from build123d import *

# Parameters (mm, degrees)
F1_DEPTH = 25
F2_DEPTH = 25
F3_R     = 10.5
F4_DEPTH = 25
F6_DEPTH = 25


with BuildPart() as f1:
    # F0 (on Top) → F1 (new body)
    with BuildSketch(Plane.XY):
        with BuildLine():
            Line((-7.459, 75), (-15, 75))
            Line((-15, 75), (-15, 15))
            ThreePointArc((-15, 15), (-16.614759, 6.882058), (-21.213203, 0))
            Line((-21.213203, 0), (-63.534251, -42.321048))
            Line((-63.534251, -42.321048), (-58.201959, -47.65334))
            Line((-58.201959, -47.65334), (-21.537765, -10.989146))
            Line((-21.537765, -10.989146), (-10.989146, -21.537765))
            Line((-10.989146, -21.537765), (-47.65334, -58.201959))
            Line((-47.65334, -58.201959), (-42.321048, -63.534251))
            Line((-42.321048, -63.534251), (0, -21.213203))
            Line((0, -21.213203), (42.321048, -63.534251))
            Line((42.321048, -63.534251), (47.65334, -58.201959))
            Line((47.65334, -58.201959), (10.989146, -21.537765))
            Line((10.989146, -21.537765), (21.537765, -10.989146))
            Line((21.537765, -10.989146), (58.201959, -47.65334))
            Line((58.201959, -47.65334), (63.534251, -42.321048))
            Line((63.534251, -42.321048), (21.213203, 0))
            ThreePointArc((21.213203, 0), (16.614759, 6.882058), (15, 15))
            Line((15, 15), (15, 75))
            Line((15, 75), (7.459, 75))
            Line((7.459, 75), (7.459, 23.149))
            Line((7.459, 23.149), (-7.459, 23.149))
            Line((-7.459, 23.149), (-7.459, 75))
        make_face()
    extrude(amount=F1_DEPTH)

    # F0 (on Top) → F2 (join)
    with BuildSketch(Plane.XY):
        with BuildLine():
            Line((-15, 15), (-15, 75))
            ThreePointArc((-15, 75), (-36.186316, 15.064984), (-63.534251, -42.321048))
            Line((-63.534251, -42.321048), (-21.213203, 0))
            ThreePointArc((-21.213203, 0), (-16.614759, 6.882058), (-15, 15))
        make_face()
        with BuildLine():
            ThreePointArc((63.534251, -42.321048), (36.207052, 15.073562), (15, 75))
            Line((15, 75), (15, 15))
            ThreePointArc((15, 15), (16.614759, 6.882058), (21.213203, 0))
            Line((21.213203, 0), (63.534251, -42.321048))
        make_face()
        with BuildLine():
            Line((0, -21.213203), (-42.321048, -63.534251))
            ThreePointArc((-42.321048, -63.534251), (0, -52.921768), (42.321048, -63.534251))
            Line((42.321048, -63.534251), (0, -21.213203))
        make_face()
    extrude(amount=F2_DEPTH)

    # F3 (on face) → F4 (cut)
    with BuildSketch(Plane.XY.offset(25)):
        Circle(F3_R)
    extrude(amount=-F4_DEPTH, mode=Mode.SUBTRACT)

    # F5 (on face) → F6 (cut)
    with BuildSketch(Plane.XY.offset(25)):
        with BuildLine():
            ThreePointArc((-15.367649, 53.450763), (-29.148649, 12.456713), (-47.984254, -26.474612))
            Line((-47.984254, -26.474612), (-21.509642, 0))
            ThreePointArc((-21.509642, 0), (-16.96133, 6.99149), (-15.367649, 15.178569))
            Line((-15.367649, 15.178569), (-15.367649, 53.450763))
        make_face()
        with BuildLine():
            ThreePointArc((-28.007545, -49.472019), (0.463168, -44.355391), (28.851137, -49.912784))
            Line((28.851137, -49.912784), (0, -21.263063))
            Line((0, -21.263063), (-28.007545, -49.472019))
        make_face()
        with BuildLine():
            ThreePointArc((47.949795, -26.474612), (29.787416, 12.835137), (14.770781, 53.450763))
            Line((14.770781, 53.450763), (14.770781, 15.619874))
            ThreePointArc((14.770781, 15.619874), (16.322077, 7.253759), (20.769704, 0))
            Line((20.769704, 0), (47.949795, -26.474612))
        make_face()
    extrude(amount=-F6_DEPTH, mode=Mode.SUBTRACT)


solid = f1.part
Geometry check sheet. Reference: the model listing, model coordinates, mm. A direction names the side the tool comes from. Give positions to 0.01 mm unless a question says otherwise; leave off trailing zeros. Order: outer loops, then holes, each group sorted by start corner. A loop starts at its lowest first (then second) coordinate and runs counter-clockwise, first axis right, second up. Notation, with made-up numbers: M 65.25,59 L 92.25,59 A17 ccw 92.25,89 Z; hole C 78.5,53.5 d3. An arc over 180 degrees is marked long. Use a Markdown table: item, result.
Item 1: Material ranges on line 1 along Y through (x, z) = (0, 11.5); line 2 along X through (y, z) = (-6, 18); line 3 along X through (y, z) = (-37, 3.75), recorded low to high.
Answers follow:
| item | result |
|---|---|
| line 1 | y = -52.92 to -44.35, -21.26 to -10.5, 10.5 to 23.15 |
| line 2 | x = -45.37 to -37.32, -27.51 to -8.62, 8.62 to 26.93, 38.02 to 45.39 |
| line 3 | x = -60.68 to -47.55, -26.45 to -15.62, 15.85 to 26.45, 47.55 to 60.69 |
Item 2: Tool access check on faces 4 (the flat face through (0, 23.149, 12)), 5 (the cylindrical face through (16.279, 7.366, 12.675)), 6 (the flat face through (60.831, -45.025, 12.325)). Record the directions out of +Z, -Z, +X, -X, +Y, -Y that give a thin tool (end or side, any length) a straight path to the whole face; none if there is none.
Answers follow:
| item | result |
|---|---|
| face 4 | +Z, -Z, +Y |
| face 5 | +Z, -Z |
| face 6 | +Z, -Z, +X, -Y |
Item 3: Draft check along Y on faces 1 (the flat face through (14.771, 35, 13)), 2 (the flat face through (-7.459, 49, 12)), 3 (the cylindrical face through (-35.847, 15.888, 12.325)). Enter one of: +Y half, -Y half, draft (parallel to the pull), parting line (faces both ways), or undercut.
Answers follow:
| item | result |
|---|---|
| face 1 | undercut |
| face 2 | draft |
| face 3 | +Y half |
Item 4: Section check A-A (y = 34.5). Record the cut outline in (x, z).
Answers follow:
| item | result |
|---|---|
| outline | M -28.54,0 L -21.02,0 L -21.02,25 L -28.54,25 Z; M -15.37,0 L -7.46,0 L -7.46,25 L -15.37,25 Z; M 7.46,0 L 14.77,0 L 14.77,25 L 7.46,25 Z; M 21.33,0 L 28.56,0 L 28.56,25 L 21.33,25 Z |
Item 5: Section check D-D (x = -45). Record the cut outline in (y, z), and give its area (3 significant figures).
Answers follow:
| item | result |
|---|---|
| outline | M -60.86,0 L -55.55,0 L -55.55,25 L -60.86,25 Z; M -34.45,0 L -23.49,0 L -23.49,25 L -34.45,25 Z; M -21.07,0 L -5.19,0 L -5.19,25 L -21.07,25 Z |
| area | 804 mm2 |
Item 6: Depth check by flat-ended pin: P1, Ø12.5, axis at y = 29.5, z = 17.5, coming from the -X side; P2, Ø10, axis at x = 45.5, y = -38.5, coming from the +Z side; P3, Ø10, axis at x = 30.5, z = 10.5, coming from the -Y side; P4, Ø10, axis at x = -17, z = 9, coming from the -Y side. Enter the tip coordinate at first touch or a pass-through.
Answers follow:
| item | result |
|---|---|
| P1 | stops at x = -32.87 |
| P2 | stops at z = 25 |
| P3 | stops at y = -60.25 |
| P4 | stops at y = -55.66 |
Item 7: Section check C-C (z = 22.5). State how many separate pieces and enclosed holes the cut face has, and give its area (3 significant figures).
Answers follow:
| item | result |
|---|---|
| separate pieces | 1 |
| enclosed holes | 4 |
| area | 5,740 mm2 |
Item 8: Section check B-B (x = -24.5). Record the cut outline in (y, z).
Answers follow:
| item | result |
|---|---|
| outline | M -56.33,0 L -48.23,0 L -48.23,25 L -56.33,25 Z; M -45.94,0 L -35.05,0 L -35.05,25 L -45.94,25 Z; M -13.95,0 L -2.99,0 L -2.99,25 L -13.95,25 Z; M 24.49,0 L 45.62,0 L 45.62,25 L 24.49,25 Z |
